Autodesk Inventor part; units mm, degrees
ref_plane "YZ Plane" through (0, 0, 0) normal (1, 0, 0) x (0, 1, 0)
ref_plane "XZ Plane" through (0, 0, 0) normal (0, 1, 0) x (-1, 0, 0)
ref_plane "XY Plane" through (0, 0, 0) normal (0, 0, 1) x (1, 0, 0)
sketch "Skizze1" plane through (0, 0, 0) normal (0, 1, 0) x (-1, 0, 0)
  line L0 (100.9437, 169.5604) -> (-41.0563, 169.5604)
  line L1 (-41.0563, 169.5604) -> (-41.0563, -140.4396)
  line L2 (-41.0563, -140.4396) -> (100.9437, -140.4396)
  line L3 (100.9437, -140.4396) -> (100.9437, 169.5604)
  point P0 (0, 0)
  dimension "d0" = 142
  dimension "d1" = 310
extrude "Extrusion1" add sketch "Skizze1" along normal blind 20
sketch "Skizze3" plane through (0, 20, 0) normal (0, 1, 0) x (1, 0, 0)
  line L0 (41.0563, -169.5604) -> (41.0563, 140.4396)
  line L1 (-100.9437, -169.5604) -> (41.0563, -169.5604)
  line L2 (41.0563, 140.4396) -> (-15.9437, 140.4396)
  line L3 (-15.9437, 140.4396) -> (-15.9437, -169.5604)
  line L4 (-15.9437, -169.5604) -> (41.0563, -169.5604)
  line L5 (41.0563, -169.5604) -> (41.0563, 140.4396)
  line L6 (-100.9437, 140.4396) -> (-100.9437, -169.5604)
  line L7 (-55.1017, 146.8416) -> (-0.3577, 14.6778)
  line L8 (0.4663, 14.6778) -> (101.62, -86.4759)
  line L9 (-0.3577, 14.6778) -> (0.4663, 14.6778)
  point P0 (0, 0)
  point P1 (-15.9437, 52.3058)
  point P2 (41.0563, -25.9122)
  dimension "d66" = 85
  dimension "d69" = 157.5
  dimension "d70" = 316.402
  dimension "d71" = 45.842
  dimension "d72" = 143.053
  dimension "d74" = 143.053
  dimension "d75" = 157.5
  dimension "d76" = 0
  dimension "d77" = 0.824
extrude "Extrusion4" cut sketch "Skizze3" against normal through all contours L8 L9 L7 L3 L2 L0
fillet "Rundung1" radius 2 4 edges at (-100.9437, 20, 14.5604) (-100.9437, 0, 14.5604) (41.0563, 20, 97.7363) (41.0563, 0, 97.7363)
properties part number "VerstaerkungHintenLinks"
Can you work these out from the model? Positions are in its coordinate system, mm. A direction names the side the tool comes from. Round coordinates to 2 decimals unless told otherwise and drop trailing zeros. Order: outer loops, then holes, each group sorted by start corner. A loop starts at its lowest first (then second) coordinate and runs counter-clockwise, first axis right, second up.
(1) If we section it at C-C (x = 28.5): Please give me the cut outline in (y, z), plus the area to 3 significant figures.
Results are:
outline: (0, 13.36) - (20, 13.36) - (20, 169.56) - (0, 169.56) - close
area: 3,120 mm2
(2) If we section it at D-D (z = -10): Please give me the cut outline in (x, y), plus the area to 3 significant figures.
Results are:
outline: (-100.94, 2) arc R2 ccw to (-98.94, 0) - (5.14, 0) - (5.14, 20) - (-98.94, 20) arc R2 ccw to (-100.94, 18) - close
area: 2,120 mm2
(3) If we section it at A-A (y = 7.75): Please give me the cut outline in (x, z).
Results are:
outline: (-100.94, -140.44) - (-15.94, -140.44) - (-15.94, -52.31) - (-0.36, -14.68) - (0.47, -14.68) - (41.06, 25.91) - (41.06, 169.56) - (-100.94, 169.56) - close
(4) If we section it at B-B (z = -86): Please give me the cut outline in (x, y).
Results are:
outline: (-100.94, 2) arc R2 ccw to (-98.94, 0) - (-15.94, 0) - (-15.94, 20) - (-98.94, 20) arc R2 ccw to (-100.94, 18) - close
(5) On a 3-axis mill with a long thin cutter (end or side, diameter ignored), from which of +Z, -Z, +X, -X, +Y, -Y can I reach the whole of each face in a straight line? I mean faces 1 (the face through (-31, 10, 169.56)), 2 (the face through (-15.944, 10, -97)). Say none if no direction works.
Results are:
face 1: +Z, +X, -X, +Y, -Y
face 2: -Z, +X, +Y, -Y
(6) I'm going to push flat-ended pins straight in: pin 1 (4 mm diameter, centred on x = -37.5, z = 15.5, fed in from -Y); pin 2 (12 mm diameter, centred on y = 14.5, z = -10.5, fed in from +X). Where does each tip first touch, or does it pass through?
Results are:
pin 1: stops at y = 0
pin 2: stops at x = 10.64
(7) If I drill on L1, parallel to X at y = 7.5, z = -123; L2, parallel to X at y = 18.5, z = 120.5; L3, parallel to Z at x = 21.5, y = 19.25, over which ranges is the centre line in solid material (lowest first)?
Results are:
L1: x = -100.94 to -15.94
L2: x = -100.88 to 40.99
L3: z = 6.36 to 169.56
